```python
from build123d import *

# Parameters (mm, degrees)
BOSS_EXTRUDE1_DEPTH = 12
SKETCH3_W           = 4.4
SKETCH3_H           = 4
CUT_REVOLVE1_ANGLE  = 3
SKETCH4_W           = 4
SKETCH4_H           = 4
REVOLVE1_ANGLE      = 3


with BuildPart() as part:
    # Sketch1 → Boss-Extrude1 (new body)
    with BuildSketch(Plane(origin=(0, 0, 0), x_dir=(1, 0, 0), z_dir=(0, 1, 0))):
        with BuildLine():
            Line((-211.174799688, 206.201137862), (-182.564973394, 178.265140079))
            ThreePointArc((-182.564973394, 178.265140079), (-212.957593109, 140.868101899), (-235.777573605, 98.424041209))
            ThreePointArc((-235.777573605, 98.424041209), (-249.780718251, 52.966609881), (-255.104275502, 5.700069272))
            Line((-255.104275502, 5.700069272), (-255.104275502, 4.568862205))
            Line((-255.104275502, 4.568862205), (-295.085665641, 4.092423829))
            Line((-295.085665641, 4.092423829), (-295.085665641, 6.176990522))
            ThreePointArc((-295.085665641, 6.176990522), (-272.171507635, 114.17694912), (-211.174799688, 206.201137862))
        make_face()
        Polygon((-288.853949055, 28.475508763), (-289.795828236, 7.496641691), (-259.297708464, 6.269015395), (-258.355829283, 27.247882467), align=None, mode=Mode.SUBTRACT)
        Polygon((-288.202969042, 34.784391797), (-257.949644018, 30.724233072), (-254.683431263, 51.47416217), (-285.407974911, 55.597560966), align=None, mode=Mode.SUBTRACT)
        Polygon((-283.612878523, 61.915838046), (-253.89939669, 54.933619681), (-248.631031599, 75.267631401), (-278.809043274, 82.359007245), align=None, mode=Mode.SUBTRACT)
        Polygon((-276.255921554, 89.176800074), (-247.361344598, 79.340855863), (-240.142390382, 99.066838813), (-269.488694715, 109.056554622), align=None, mode=Mode.SUBTRACT)
        Polygon((-230.355302506, 120.079310533), (-239.303938624, 101.075373705), (-267.042878446, 114.91557665), (-257.667257096, 133.706471368), align=None, mode=Mode.SUBTRACT)
        Polygon((-217.599523923, 141.890991255), (-228.352118631, 123.846340791), (-254.61522008, 140.315994772), (-243.458357706, 158.107128012), align=None, mode=Mode.SUBTRACT)
        Polygon((-203.234989184, 161.794735755), (-215.691212171, 144.88112549), (-240.228428406, 163.826442046), (-227.39588109, 180.449490275), align=None, mode=Mode.SUBTRACT)
        Polygon((-186.795494279, 179.950119438), (-201.048962764, 164.528101536), (-223.368087677, 185.348741273), (-209.114619192, 200.770759174), align=None, mode=Mode.SUBTRACT)
    extrude(amount=BOSS_EXTRUDE1_DEPTH)

    # Sketch3 → Cut-Revolve1 (revolve, cut)
    with BuildSketch(Plane(origin=(-0.090657576, 0, -7.607732879), x_dir=(0.9999290060329473, 0, -0.01191565751279397), z_dir=(0.01191565751279397, 0, 0.9999290060329473))):
        with Locations((-256.83172364, 6.020050252)):
            Rectangle(SKETCH3_W, SKETCH3_H)
        with Locations((-293.215952418, 6.020050252)):
            Rectangle(SKETCH3_W, SKETCH3_H)
    revolve(axis=Axis((-0.090657576, 0, -7.607732879), (0, -1, 0)), revolution_arc=CUT_REVOLVE1_ANGLE, mode=Mode.SUBTRACT)

    # Sketch4 → Revolve1 (revolve)
    with BuildSketch(Plane(origin=(0, 0, 0), x_dir=(-0.715482223100618, 0, -0.6986309386414242), z_dir=(0.6986309386414242, 0, -0.715482223100618))):
        with Locations((257.163535165, 6)):
            Rectangle(SKETCH4_W, SKETCH4_H)
        with Locations((293.150309637, 6)):
            Rectangle(SKETCH4_W, SKETCH4_H)
    revolve(axis=Axis((0, 0, 0), (0, -1, 0)), revolution_arc=REVOLVE1_ANGLE)


solid = part.part
```
CAD build for the part. Positions are in the model's coordinates, mm. A direction names the side the tool comes from. Coordinates: 2 decimals unless noted, no trailing zeros. Write each loop counter-clockwise with the first axis right and the second up, starting at its lowest first coordinate (ties: lowest second). Pieces come first, ordered by that corner, then holes. Notation, with made-up numbers: (76.25, 45) -> (83.25, 45) arc R29 ccw to (83.25, 74) -> close; hole circle Ø5 at (64.5, -16.75). An arc over 180 degrees is marked (long way). Return JSON: item names as keys, results as strings. Group by question number.
Q1. Cut at C-C, the plane z = -128.5. Give the cut face in (x, y) (3 decimals), then the cut area to 3 significant figures.
Q2. Pull direction X, two halves, no side cores. Call faces 4 (the face through (-293, 8.02, -12)), 5 (the face through (-243.8, 5.92, -89.07)), 6 (the face through (-177.9, 6.03, -182.92)): released by +X, released by -X, zero draft, split by the parting line, or undercut.
Q3. Cut at B-B, the plane x = -273. Give the cut face in (y, z), then the cut area to 3 significant figures.
Q4. Flat gauge pins, fed straight in: pin 1 (15 mm diameter, centred on x = -202.5, z = -212, fed in from +Y); pin 2 (2.5 mm diameter, centred on x = -256, z = -9.5, fed in from -Y); pin 3 (11 mm diameter, centred on x = -203.5, z = -208.5, fed in from -Y); pin 4 (0.9 mm diameter, centred on y = 2.5, z = -5.5, fed in from +X). Where does each tip first touch, or does it go through?
Q5. Cut at A-A, the plane z = -195.5. Give the cut face in (x, y).
Q6. Drill centre lines: line 1 (Z direction, x = -204.5, y = 5.5); line 2 (Z direction, x = -199, y = 5); line 3 (X direction, y = 4, z = -127.5). Where is each one in solid material? Low to high.
Q7. Which spindle directions (+Z, -Z, +X, -X, +Y, -Y) get a long thin tool onto all of the face, cutting with end or side? Do faces 1 (the face through (-256.7, 6.05, -17.99)), 2 (the face through (-179, 8, -184)), 3 (the face through (-256.34, 5.92, -40.95)). Say none if no direction does.
Q8. Cut at D-D, the plane y = 2. State how many separate pieces and enclosed holes the cut face has, then the cut area to 3 significant figures.
Returned:
{
 "1": {"outline": "(-265.709, 0) -> (-260.265, 0) -> (-260.265, 12) -> (-265.709, 12) -> close; (-247.232, 0) -> (-235.773, 0) -> (-235.773, 12) -> (-247.232, 12) -> close; (-225.579, 0) -> (-220.699, 0) -> (-220.699, 12) -> (-225.579, 12) -> close", "area": "261 mm2"},
 "2": {"face 4": "zero draft", "face 5": "undercut", "face 6": "released by +X"},
 "3": {"outline": "(0, -112.18) -> (12, -112.18) -> (12, -98.74) -> (0, -98.74) -> close; (0, -88.07) -> (12, -88.07) -> (12, -80.99) -> (0, -80.99) -> close; (0, -59.42) -> (12, -59.42) -> (12, -53.93) -> (0, -53.93) -> close; (0, -32.74) -> (12, -32.74) -> (12, -27.84) -> (0, -27.84) -> close; (0, -6.82) -> (12, -6.82) -> (12, -4.36) -> (0, -4.36) -> close", "area": "401 mm2"},
 "4": {"pin 1": "stops at y = 8", "pin 2": "stops at y = 0", "pin 3": "stops at y = 4", "pin 4": "stops at x = -255.1"},
 "5": {"outline": "(-221.12, 0) -> (-213.99, 0) -> (-213.99, 12) -> (-221.12, 12) -> close; (-203.46, 0) -> (-200.22, 0) -> (-200.22, 12) -> (-203.46, 12) -> close"},
 "6": {"line 1": "z = -212.82 to -207.24, -199.68 to -196.47, -167.75 to -162.77, -160.08 to -152.8", "line 2": "z = -215.78 to -212.53, -194.31 to -191.34, -166.75 to -159.85", "line 3": "x = -266.19 to -260.76, -245.23 to -234.18, -226.17 to -221.28"},
 "7": {"face 1": "+Z", "face 2": "-Z, +X, +Y", "face 3": "+Y, -Y"},
 "8": {"separate pieces": "1", "enclosed holes": "8", "area": "3,150 mm2"}
}
